Autodesk Inventor part; units mm, degrees
ref_plane "YZ Plane" through (0, 0, 0) normal (1, 0, 0) x (0, 1, 0)
ref_plane "XZ Plane" through (0, 0, 0) normal (0, 1, 0) x (-1, 0, 0)
ref_plane "XY Plane" through (0, 0, 0) normal (0, 0, 1) x (1, 0, 0)
sketch "Sketch1" plane through (0, 0, 0) normal (0, 0, 1) x (1, 0, 0)
  line L0 (0, 0) -> (38, 0)
  line L1 (38, 0) -> (38, 61)
  line L2 (38, 61) -> (0, 61)
  line L3 (0, 61) -> (0, 0)
  line L4 (0, 61) -> (4, 61)
  line L5 (4, 61) -> (4, 55)
  line L6 (38, 61) -> (34, 61)
  line L7 (34, 61) -> (34, 55)
  line L8 (38, 0) -> (34, 0)
  line L9 (34, 0) -> (34, 4.5)
  line L10 (0, 0) -> (4, 0)
  line L11 (4, 0) -> (4, 4.5)
  circle A0 centre (4, 4.5) radius 1.5
  circle A1 centre (34, 4.5) radius 1.5
  circle A2 centre (34, 55) radius 1.5
  circle A3 centre (4, 55) radius 1.5
  dimension "d0" = 38
  dimension "d1" = 61
  dimension "d2" = 4
  dimension "d3" = 6
  dimension "d4" = 4
  dimension "d5" = 6
  dimension "d6" = 4
  dimension "d7" = 4.5
  dimension "d8" = 4
  dimension "d9" = 4.5
  dimension "d10" = 3
  dimension "d11" = 3
  dimension "d12" = 3
  dimension "d13" = 3
extrude "Extrusion1" add sketch "Sketch1" along normal blind 5
sketch "Sketch2" plane through (0, 0, 5) normal (0, 0, 1) x (1, 0, 0)
  line L0 (38, 61) -> (0, 61)
  line L1 (0, 61) -> (3, 61)
  line L2 (3, 61) -> (3, 42.5)
  line L3 (3, 42.5) -> (12, 42.5)
  line L4 (12, 42.5) -> (12, 28.5)
  line L5 (12, 28.5) -> (3, 28.5)
  line L6 (3, 28.5) -> (3, 42.5)
  line L7 (3, 42.5) -> (3, 51.2798)
  point P0 (0, 0)
  dimension "d16" = 3
  dimension "d17" = 18.5
  dimension "d18" = 9
  dimension "d19" = 14
  dimension "d20" = 9
extrude "Extrusion2" cut sketch "Sketch2" against normal through all
properties part number "arm_1_case"
Can you work these out from the model? Positions are in its coordinate system, mm. A direction names the side the tool comes from. Give positions to 0.01 mm unless a question says otherwise; leave off trailing zeros. Write each loop counter-clockwise with the first axis right and the second up, starting at its lowest first coordinate (ties: lowest second). Pieces come first, ordered by that corner, then holes. Notation, with made-up numbers: (8.5, 14) - (20.5, 14) arc R11 ccw to (20.5, 29) - close; hole circle Ø10 at (72, -23). An arc over 180 degrees is marked (long way). Write item = value, one per line. Start each with the question number.
1. On a 3-axis mill with a long thin cutter (end or side, diameter ignored), from which of +Z, -Z, +X, -X, +Y, -Y can I reach the whole of each face in a straight line? I mean faces 4 (the face through (19, 31, 5)), 5 (the face through (7, 42.5, 3)). Say none if no direction works.
2. Imagine slicing it at B-B (x = 34). Please give me the cut outline in (y, z), and give its area (3 significant figures).
3. Please list where these lines run through material, in increasing order: line 1 (X direction, y = 4.5, z = 2.55); line 2 (Y direction, x = 4, z = 1.7); line 3 (Y direction, x = 34, z = 3.7).
4. Imagine slicing it at C-C (y = 55). Please give me the cut outline in (x, z), and give its area (3 significant figures).
5. Thinking about a two-plate mould opening in X: for faces 1 (the face through (32.8, 5.4, 2.5)), 2 (the face through (0, 31, 2)), 3 (the face through (19, 31, 0)), which applies, released by +X, released by -X, zero draft, split by the parting line, or undercut?
6. Imagine slicing it at A-A (z = 3.4). Please give me the cut outline in (x, y).
Worked answers:
q1.face_4 = +Z, +X, -X, +Y, -Y
q1.face_5 = +Z, -Z
q2.outline = (0, 0) - (3, 0) - (3, 5) - (0, 5) - close; (6, 0) - (53.5, 0) - (53.5, 5) - (6, 5) - close; (56.5, 0) - (61, 0) - (61, 5) - (56.5, 5) - close
q2.area = 275 mm2
q3.line_1 = 0 to 2.5, 5.5 to 32.5, 35.5 to 38
q3.line_2 = 0 to 3, 6 to 28.5, 42.5 to 53.5, 56.5 to 61
q3.line_3 = 0 to 3, 6 to 53.5, 56.5 to 61
q4.outline = (0, 0) - (2.5, 0) - (2.5, 5) - (0, 5) - close; (5.5, 0) - (32.5, 0) - (32.5, 5) - (5.5, 5) - close; (35.5, 0) - (38, 0) - (38, 5) - (35.5, 5) - close
q4.area = 160 mm2
q5.face_1 = undercut
q5.face_2 = released by -X
q5.face_3 = zero draft
q6.outline = (0, 0) - (38, 0) - (38, 61) - (0, 61) - close; hole circle Ø3 at (4, 4.5); hole circle Ø3 at (4, 55); hole (3, 28.5) - (12, 28.5) - (12, 42.5) - (3, 42.5) - close; hole circle Ø3 at (34, 4.5); hole circle Ø3 at (34, 55)
